For this review, use the dimensioned drawing (mm, ordinates from the lowest corner) and the shaded views. A direction names the side the tool comes from. Coordinates: 2 decimals unless noted, no trailing zeros. Loops run counter-clockwise (first coordinate to the right, second up) from the corner with the lowest first, then second, coordinate; pieces in that order, holes last. Notation, with made-up numbers: (-36.75, 34.25) - (19.25, 34.25) arc R9 cw to (19.25, 48.25) - close; hole circle Ø11 at (22.5, 84). An arc over 180 degrees is marked (long way). Answer in a Markdown table with one row per item. Add a question column.
(1) Machinability: for the marked faces 1, 2 and 3, which of the approach directions +Z, -Z, +X, -X, +Y, -Y give a long, thin tool a straight path to every point of the face, cutting with its end or side? Answer none if there is none.
(2) For line 1 along Y through (x, z) = (5.5, 2.25); line 2 along Z through (x, y) = (15, 7); line 3 along Y through (x, z) = (5.5, 4.75), list the stretches that pass through material, from the lowest coordinate up.
(3) We need section C-C on y = 6.5. Write out the cut boundary in (x, z), plus the area to 3 significant figures.
(4) Mouldability with a two-part tool opening along X and no side actions: class the marked faces 4, 5 and 6 as +X half, -X half, draft (parallel to the pull), parting line (faces both ways), or undercut.
(5) We need section B-B on z = 5. Write out the cut boundary in (x, y), plus the area to 3 significant figures.
(6) For P1, Ø1.1, axis at x = 6.5, y = 0.5, coming from the -Z side; P2, Ø4, axis at x = 7, z = 1.5, coming from the -Y side; P3, Ø2.5, axis at x = 16.5, z = 6, coming from the +Y side; P4, Ø0.8, axis at x = 18.5, y = 0.5, coming from the +Z side, all flat-tipped, find the tip position at first contact; note any pin that passes through.
(7) We need section D-D on z = 9. Write out the cut boundary in (x, y).
(8) We need section A-A on x = 5.5. Write out the cut boundary in (y, z).
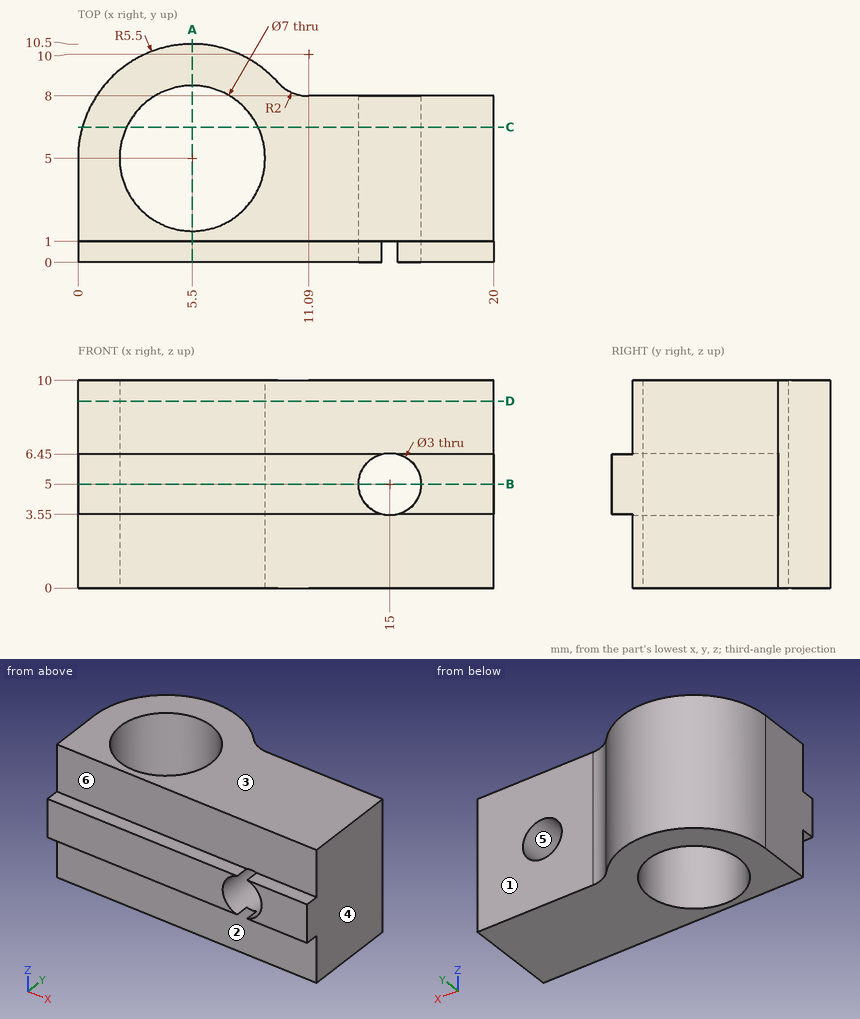
Outcome:
| question | item | result |
|---|---|---|
| 1 | face 1 | +Z, -Z, +X, +Y |
| 1 | face 2 | -Z, +X, -X, -Y |
| 1 | face 3 | +Z, +X, -X, +Y, -Y |
| 2 | line 1 | 1 to 1.5, 8.5 to 10.5 |
| 2 | line 2 | 0 to 3.5, 6.5 to 10 |
| 2 | line 3 | 0 to 1.5, 8.5 to 10.5 |
| 3 | outline | (0.21, 0) - (2.34, 0) - (2.34, 10) - (0.21, 10) - close; (8.66, 0) - (20, 0) - (20, 10) - (8.66, 10) - close; hole circle Ø3 at (15, 5) |
| 3 | area | 128 mm² |
| 4 | face 4 | +X half |
| 4 | face 5 | undercut |
| 4 | face 6 | draft |
| 5 | outline | (0, 0) - (13.5, 0) - (13.5, 8) - (11.09, 8) arc R2 cw to (9.6, 8.67) arc R5.5 ccw to (0, 5) - close; (16.5, 0) - (20, 0) - (20, 8) - (16.5, 8) - close; hole circle Ø7 at (5.5, 5) |
| 5 | area | 113 mm² |
| 6 | P1 | z = 0 |
| 6 | P2 | y = 1 |
| 6 | P3 | y = 8 |
| 6 | P4 | z = 6.45 |
| 7 | outline | (0, 1) - (20, 1) - (20, 8) - (11.09, 8) arc R2 cw to (9.6, 8.67) arc R5.5 ccw to (0, 5) - close; hole circle Ø7 at (5.5, 5) |
| 8 | outline | (0, 3.55) - (1, 3.55) - (1, 0) - (1.5, 0) - (1.5, 10) - (1, 10) - (1, 6.45) - (0, 6.45) - close; (8.5, 0) - (10.5, 0) - (10.5, 10) - (8.5, 10) - close |
